Part print with two shaded views. Sizes in mm from the minimum x, y, z corner. A direction names the side the tool comes from. Coordinates: 2 decimals unless noted, no trailing zeros. Loops run counter-clockwise (first coordinate to the right, second up) from the corner with the lowest first, then second, coordinate; pieces in that order, holes last. Notation, with made-up numbers: (49.25, 27) - (90.25, 27) arc R24 cw to (90.25, 64) - close; hole circle Ø8 at (-32.5, 69). An arc over 180 degrees is marked (long way). Write each question's results on one line, items separated by ' | '. Start each with the question number.
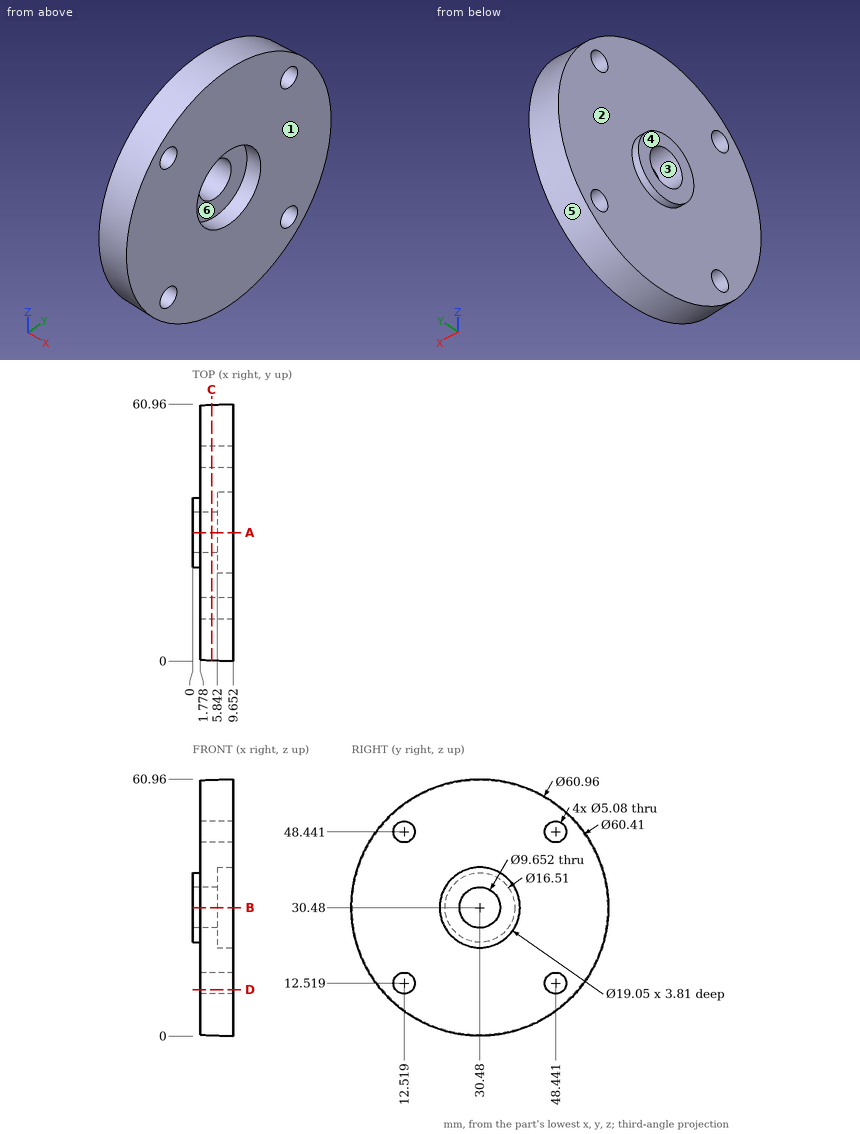
Q1. Which spindle directions (+Z, -Z, +X, -X, +Y, -Y) get a long thin tool onto all of the face, cutting with end or side? Do the marked faces 1 and 2. Say none if no direction does.
Q2. Mould opens along Z. For the marked faces 3, 4, 5 and 6 say: +Z half, -Z half, draft (parallel to the pull), parting line (faces both ways), or undercut.
Q3. Cut at D-D (z = 11). State how many separate pieces and enclosed holes the cut face has, and give its area (3 significant figures).
Q4. Cut at C-C (x = 4.5). List the corners of the cut face in (y, z).
Q5. Pin check, flat tips, straight feed: pin 1 (3 mm diameter, centred on x = 4, y = 31.5, fed in from -Z); pin 2 (6.5 mm diameter, centred on y = 48.44, z = 12.52, fed in from -X); pin 3 (5 mm diameter, centred on x = 5.5, y = 9, fed in from -Z). Stop position of each tip, or through.
Q6. Drill centre lines: L1, parallel to Z at x = 4.75, y = 10.5; L2, parallel to X at y = 42.5, z = 39; L3, parallel to Y at x = 7, z = 13.5 (1 decimal). Where is each one in solid material? Low to high. Write a range as from..to.
Q7. Cut at A-A (y = 30.48). List the corners of the cut face in (x, z) (1 decimal).
Check result:
1) face 1: +Z, -Z, +X, +Y, -Y | face 2: -X
2) face 3: undercut | face 4: draft | face 5: parting line | face 6: undercut
3) separate pieces: 3 | enclosed holes: 0 | area: 302 mm²
4) outline: circle Ø60.6 at (30.48, 30.48); hole circle Ø5.08 at (12.52, 12.52); hole circle Ø5.08 at (12.52, 48.44); hole circle Ø9.65 at (30.48, 30.48); hole circle Ø5.08 at (48.44, 12.52); hole circle Ø5.08 at (48.44, 48.44)
5) pin 1: z = 0.15 | pin 2: x = 1.78 | pin 3: z = 6.81
6) L1: 7.69..10.98, 14.06..46.9, 49.98..53.27 | L2: 1.78..9.65 | L3: 5.3..10.2, 14.9..46.1, 50.8..55.7
7) outline: (0, 22.2) - (1.8, 22.2) - (1.8, 0.3) - (9.7, 0) - (9.7, 21) - (5.8, 21) - (5.8, 25.7) - (0, 25.7) - close; (0, 35.3) - (5.8, 35.3) - (5.8, 40) - (9.7, 40) - (9.7, 61) - (1.8, 60.7) - (1.8, 38.7) - (0, 38.7) - close
